Check sheet for the drawn part. Datum: minimum x, y, z corner. Units: mm. A direction names the side the tool comes from. Give positions to 0.01 mm unless a question says otherwise; leave off trailing zeros. Write each loop counter-clockwise with the first axis right and the second up, starting at its lowest first coordinate (ties: lowest second). Pieces come first, ordered by that corner, then holes. Notation, with made-up numbers: (-7, 17.25) -> (50, 17.25) arc R20 cw to (50, 52.25) -> close; hole circle Ø1 at (-5.75, -25). An arc over 180 degrees is marked (long way). Answer as CSV lines item,"result". Start each with the question number.
1) Mould release check, pull along Z, two halves, no side actions. Record for the marked faces 1, 2 and 3: released by +Z, released by -Z, zero draft, split by the parting line, or undercut.
2) Sectioned sample at B-B on x = 131. Record the cut outline in (y, z) (1 decimal).
3) Tool access check on the marked faces 4 and 5. Record the directions out of +Z, -Z, +X, -X, +Y, -Y that give a thin tool (end or side, any length) a straight path to the whole face; none if there is none.
4) Sectioned sample at D-D on y = 64.5. Record the cut outline in (x, z), and give its area (3 significant figures).
5) Sectioned sample at C-C on z = 75. Record the cut outline in (x, y) (1 decimal).
6) Gauge pin test, flat ends, axial feed: pin 1 Ø1.5 at (x, z) = (100, 45.5) entering from -Y; pin 2 Ø8 at (x, y) = (69.5, 41) entering from -Z; pin 3 Ø2 at (x, y) = (48, 36.5) entering from +Z; pin 4 Ø8 at (y, z) = (68, 133) entering from +X. Record the tip position at first contact, or that the pin passes through.
7) Sectioned sample at A-A on x = 75. Record the cut outline in (y, z), and give its area (3 significant figures).
8) Material ranges on L1, parallel to Y at x = 13.5, z = 71; L2, parallel to X at y = 64, z = 69.5; L3, parallel to X at y = 4, z = 118.5 (1 decimal), recorded low to high.
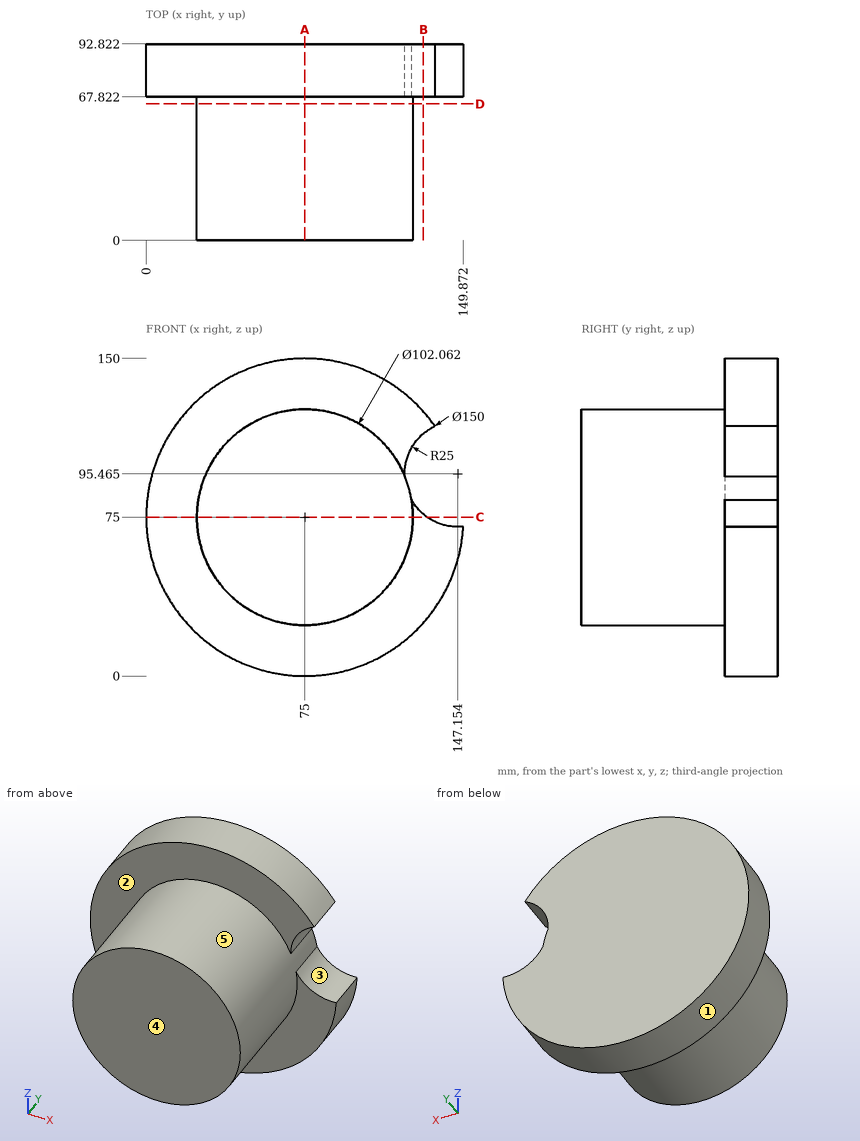
Ans:
1,face 1,"split by the parting line"
1,face 2,"zero draft"
1,face 3,"undercut"
2,outline,"(67.8, 25.1) -> (92.8, 25.1) -> (92.8, 76.4) -> (67.8, 76.4) -> close; (67.8, 114.5) -> (92.8, 114.5) -> (92.8, 124.9) -> (67.8, 124.9) -> close"
3,face 4,"+Z, -Z, +X, -X, -Y"
3,face 5,"-Y"
4,outline,"circle Ø102.06 at (75, 75)"
4,area,"8,180 mm²"
5,outline,"(0, 67.8) -> (24, 67.8) -> (24, 0) -> (126, 0) -> (126, 67.8) -> (132.8, 67.8) -> (132.8, 92.8) -> (0, 92.8) -> close"
6,pin 1,"stops at y = 0"
6,pin 2,"stops at z = 23.99"
6,pin 3,"stops at z = 118.91"
6,pin 4,"stops at x = 127.05"
7,outline,"(0, 23.97) -> (67.82, 23.97) -> (67.82, 0) -> (92.82, 0) -> (92.82, 150) -> (67.82, 150) -> (67.82, 126.03) -> (0, 126.03) -> close"
7,area,"10,700 mm²"
8,L1,"y = 67.82 to 92.82"
8,L2,"x = 24.27 to 125.73"
8,L3,"x = 48.3 to 101.7"
